Verification items for the finished model (mm, model axes). Round coordinates to 2 decimals unless told otherwise and drop trailing zeros. Write each loop counter-clockwise with the first axis right and the second up, starting at its lowest first coordinate (ties: lowest second). Pieces come first, ordered by that corner, then holes.
Autodesk Inventor part; units mm, degrees
ref_plane "YZ Plane" through (0, 0, 0) normal (1, 0, 0) x (0, 1, 0)
ref_plane "XZ Plane" through (0, 0, 0) normal (0, 1, 0) x (-1, 0, 0)
ref_plane "XY Plane" through (0, 0, 0) normal (0, 0, 1) x (1, 0, 0)
sketch "Sketch1" plane through (0, 0, 0) normal (0, 1, 0) x (-1, 0, 0)
  line L0 (0, 0) -> (10, 0)
  line L1 (10, -10) -> (10, -45)
  line L2 (10, -45) -> (0, -45)
  line L3 (0, -45) -> (0, 0)
  line L4 (0, 0) -> (25, 0)
  line L5 (25, 0) -> (25, -10)
  line L6 (25, -10) -> (10, -10)
  line L7 (0, -10) -> (0, 0)
  dimension "d0" = 10
  dimension "d1" = 45
  dimension "d3" = 10
  dimension "d6" = 25
extrude "Extrusion1" add sketch "Sketch1" along normal blind 3
sketch "Sketch2" plane through (0, 3, 0) normal (0, 1, 0) x (1, 0, 0)
  line L0 (0, 45) -> (-10, 45) construction
  line L1 (-10, 45) -> (0, 35) construction
  line L2 (0, 0) -> (0, 45) construction
  line L3 (0, 45) -> (-10, 35) construction
  line L4 (-10, 45) -> (-10, 10) construction
  circle A0 centre (-5, 40) radius 1.5
  dimension "d7" = 135
  dimension "d8" = 45
  dimension "d9" = 3
extrude "Extrusion2" cut sketch "Sketch2" against normal blind 10
properties part number "makerbeam_L-bracket" material "Acetal Resin, Black"
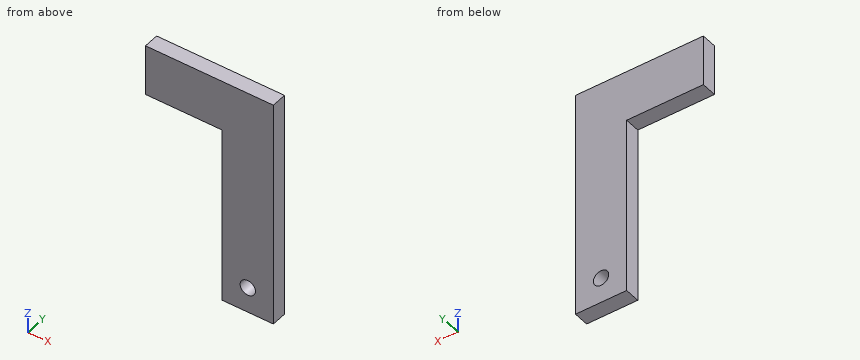
Q1. Sectioned sample at A-A (z = -40). Enter the section's corners in (x, y), plus the area to 3 significant figures.
Recorded:
outline: (-10, 0) - (-6.5, 0) - (-6.5, 3) - (-10, 3) - close; (-3.5, 0) - (0, 0) - (0, 3) - (-3.5, 3) - close
area: 21.0 mm2
Q2. Material ranges on line 1 along Z through (x, y) = (-5, 1.9); line 2 along X through (y, z) = (1.45, -40); line 3 along Z through (x, y) = (-21.5, 0.85), recorded low to high.
Recorded:
line 1: z = -45 to -41.5, -38.5 to 0
line 2: x = -10 to -6.5, -3.5 to 0
line 3: z = -10 to 0
Q3. Depth check by flat-ended pin: P1, Ø2.5, axis at x = -5, z = -40, coming from the +Y side; P2, Ø1.5, axis at y = 1.5, z = -28, coming from the -X side; P3, Ø1, axis at x = -21, y = 1.5, coming from the -Z side. Enter the tip coordinate at first touch or a pass-through.
Recorded:
P1: passes through
P2: stops at x = -10
P3: stops at z = -10
Q4. Sectioned sample at D-D (x = -21.25). Enter the section's corners in (y, z), plus the area to 3 significant figures.
Recorded:
outline: (0, -10) - (3, -10) - (3, 0) - (0, 0) - close
area: 30.0 mm2
Q5. Sectioned sample at C-C (x = -5). Enter the section's corners in (y, z).
Recorded:
outline: (0, -45) - (3, -45) - (3, -41.5) - (0, -41.5) - close; (0, -38.5) - (3, -38.5) - (3, 0) - (0, 0) - close
Q6. Sectioned sample at B-B (y = 1.5). Enter the section's corners in (x, z).
Recorded:
outline: (-25, -10) - (-10, -10) - (-10, -45) - (0, -45) - (0, 0) - (-25, 0) - close; hole circle Ø3 at (-5, -40)
